The listing builds one solid part. Answer for the finished solid, in the listing's coordinates (mm). A direction names the side the tool comes from. Coordinates: 2 decimals unless noted, no trailing zeros. Write each loop counter-clockwise with the first axis right and the second up, starting at its lowest first coordinate (ties: lowest second). Pieces come first, ordered by that corner, then holes.
from build123d import *

# Parameters (mm, degrees)
F0_R     = 3
F0_W     = 19
F0_H     = 1.5
F0_R_2   = 1
F0_W_2   = 1.5
F0_H_2   = 17.5
F0_H_3   = 11.5
F0_W_3   = 11.5
F0_W_4   = 8.5
F0_W_5   = 4.1
F1_DEPTH = 1.5
F2_DEPTH = 3
F3_DEPTH = 8
F4_DEPTH = 4.5
F5_R     = 1
F6_DEPTH = 1.5


with BuildPart() as f1:
    # F0 (on Top) → F1 (new body)
    with BuildSketch(Plane.XY):
        with BuildLine():
            Line((29.7, 15.2), (-29.7, 15.2))
            ThreePointArc((-29.7, 15.2), (-31.8213203436, 14.3213203436), (-32.7, 12.2))
            Line((-32.7, 12.2), (-32.7, 7.65))
            Line((-32.7, 7.65), (-32.7, -3.85))
            Line((-32.7, -3.85), (-32.7, -12.2))
            ThreePointArc((-32.7, -12.2), (-31.8213203436, -14.3213203436), (-29.7, -15.2))
            Line((-29.7, -15.2), (-25.85, -15.2))
            Line((-25.85, -15.2), (-14.35, -15.2))
            Line((-14.35, -15.2), (4.65, -15.2))
            Line((4.65, -15.2), (13.15, -15.2))
            Line((13.15, -15.2), (17.25, -15.2))
            Line((17.25, -15.2), (25.75, -15.2))
            Line((25.75, -15.2), (29.7, -15.2))
            ThreePointArc((29.7, -15.2), (31.8213203436, -14.3213203436), (32.7, -12.2))
            Line((32.7, -12.2), (32.7, -8.75))
            Line((32.7, -8.75), (32.7, 8.75))
            Line((32.7, 8.75), (32.7, 12.2))
            ThreePointArc((32.7, 12.2), (31.8213203436, 14.3213203436), (29.7, 15.2))
        make_face()
        with Locations((-29, -11.5)):
            Circle(F0_R, mode=Mode.SUBTRACT)
        with Locations((29, -11.5)):
            Circle(F0_R, mode=Mode.SUBTRACT)
        with Locations((-29, 11.5)):
            Circle(F0_R, mode=Mode.SUBTRACT)
        with Locations((29, 11.5)):
            Circle(F0_R, mode=Mode.SUBTRACT)
        with BuildLine():
            ThreePointArc((-32.7, 12.2), (-31.8213203436, 14.3213203436), (-29.7, 15.2))
            Line((-29.7, 15.2), (29.7, 15.2))
            ThreePointArc((29.7, 15.2), (31.8213203436, 14.3213203436), (32.7, 12.2))
            Line((32.7, 12.2), (32.7, 8.75))
            Line((32.7, 8.75), (34.2, 8.75))
            Line((34.2, 8.75), (34.2, 13.7))
            ThreePointArc((34.2, 13.7), (33.3213203436, 15.8213203436), (31.2, 16.7))
            Line((31.2, 16.7), (-31.2, 16.7))
            ThreePointArc((-31.2, 16.7), (-33.3213203436, 15.8213203436), (-34.2, 13.7))
            Line((-34.2, 13.7), (-34.2, 7.65))
            Line((-34.2, 7.65), (-32.7, 7.65))
            Line((-32.7, 7.65), (-32.7, 12.2))
        make_face()
        with BuildLine():
            Line((-32.7, -12.2), (-32.7, -3.85))
            Line((-32.7, -3.85), (-34.2, -3.85))
            Line((-34.2, -3.85), (-34.2, -13.7))
            ThreePointArc((-34.2, -13.7), (-33.3213203436, -15.8213203436), (-31.2, -16.7))
            Line((-31.2, -16.7), (-25.85, -16.7))
            Line((-25.85, -16.7), (-25.85, -15.2))
            Line((-25.85, -15.2), (-29.7, -15.2))
            ThreePointArc((-29.7, -15.2), (-31.8213203436, -14.3213203436), (-32.7, -12.2))
        make_face()
        with Locations((-4.85, -15.95)):
            Rectangle(F0_W, F0_H)
        with Locations((-29, -11.5)):
            Circle(F0_R)
        with Locations((-29, -11.5)):
            Circle(F0_R_2, mode=Mode.SUBTRACT)
        with Locations((-29, 11.5)):
            Circle(F0_R)
        with Locations((-29, 11.5)):
            Circle(F0_R_2, mode=Mode.SUBTRACT)
        with Locations((29, -11.5)):
            Circle(F0_R)
        with Locations((29, -11.5)):
            Circle(F0_R_2, mode=Mode.SUBTRACT)
        with Locations((29, 11.5)):
            Circle(F0_R)
        with Locations((29, 11.5)):
            Circle(F0_R_2, mode=Mode.SUBTRACT)
        with Locations((33.45, 0)):
            Rectangle(F0_W_2, F0_H_2)
        with BuildLine():
            Line((34.2, -8.75), (32.7, -8.75))
            Line((32.7, -8.75), (32.7, -12.2))
            ThreePointArc((32.7, -12.2), (31.8213203436, -14.3213203436), (29.7, -15.2))
            Line((29.7, -15.2), (25.75, -15.2))
            Line((25.75, -15.2), (25.75, -16.7))
            Line((25.75, -16.7), (31.2, -16.7))
            ThreePointArc((31.2, -16.7), (33.3213203436, -15.8213203436), (34.2, -13.7))
            Line((34.2, -13.7), (34.2, -8.75))
        make_face()
        with Locations((-33.45, 1.9)):
            Rectangle(F0_W_2, F0_H_3)
        with Locations((-20.1, -15.95)):
            Rectangle(F0_W_3, F0_H)
        with Locations((21.5, -15.95)):
            Rectangle(F0_W_4, F0_H)
        with Locations((8.9, -15.95)):
            Rectangle(F0_W_4, F0_H)
        with Locations((15.2, -15.95)):
            Rectangle(F0_W_5, F0_H)
        with Locations((-29, -11.5)):
            Circle(F0_R_2)
        with Locations((-29, 11.5)):
            Circle(F0_R_2)
        with Locations((29, -11.5)):
            Circle(F0_R_2)
        with Locations((29, 11.5)):
            Circle(F0_R_2)
    extrude(amount=-F1_DEPTH)

    # F0 (on Top) → F2 (join)
    with BuildSketch(Plane.XY):
        with Locations((-29, 11.5)):
            Circle(F0_R)
        with Locations((-29, 11.5)):
            Circle(F0_R_2, mode=Mode.SUBTRACT)
        with Locations((-29, -11.5)):
            Circle(F0_R)
        with Locations((-29, -11.5)):
            Circle(F0_R_2, mode=Mode.SUBTRACT)
        with Locations((29, 11.5)):
            Circle(F0_R)
        with Locations((29, 11.5)):
            Circle(F0_R_2, mode=Mode.SUBTRACT)
        with Locations((29, -11.5)):
            Circle(F0_R)
        with Locations((29, -11.5)):
            Circle(F0_R_2, mode=Mode.SUBTRACT)
    extrude(amount=F2_DEPTH)

    # F0 (on Top) → F3 (join)
    with BuildSketch(Plane.XY):
        with BuildLine():
            Line((-32.7, -12.2), (-32.7, -3.85))
            Line((-32.7, -3.85), (-34.2, -3.85))
            Line((-34.2, -3.85), (-34.2, -13.7))
            ThreePointArc((-34.2, -13.7), (-33.3213203436, -15.8213203436), (-31.2, -16.7))
            Line((-31.2, -16.7), (-25.85, -16.7))
            Line((-25.85, -16.7), (-25.85, -15.2))
            Line((-25.85, -15.2), (-29.7, -15.2))
            ThreePointArc((-29.7, -15.2), (-31.8213203436, -14.3213203436), (-32.7, -12.2))
        make_face()
        with BuildLine():
            ThreePointArc((-32.7, 12.2), (-31.8213203436, 14.3213203436), (-29.7, 15.2))
            Line((-29.7, 15.2), (29.7, 15.2))
            ThreePointArc((29.7, 15.2), (31.8213203436, 14.3213203436), (32.7, 12.2))
            Line((32.7, 12.2), (32.7, 8.75))
            Line((32.7, 8.75), (34.2, 8.75))
            Line((34.2, 8.75), (34.2, 13.7))
            ThreePointArc((34.2, 13.7), (33.3213203436, 15.8213203436), (31.2, 16.7))
            Line((31.2, 16.7), (-31.2, 16.7))
            ThreePointArc((-31.2, 16.7), (-33.3213203436, 15.8213203436), (-34.2, 13.7))
            Line((-34.2, 13.7), (-34.2, 7.65))
            Line((-34.2, 7.65), (-32.7, 7.65))
            Line((-32.7, 7.65), (-32.7, 12.2))
        make_face()
        with Locations((-4.85, -15.95)):
            Rectangle(F0_W, F0_H)
        with Locations((15.2, -15.95)):
            Rectangle(F0_W_5, F0_H)
        with BuildLine():
            Line((34.2, -8.75), (32.7, -8.75))
            Line((32.7, -8.75), (32.7, -12.2))
            ThreePointArc((32.7, -12.2), (31.8213203436, -14.3213203436), (29.7, -15.2))
            Line((29.7, -15.2), (25.75, -15.2))
            Line((25.75, -15.2), (25.75, -16.7))
            Line((25.75, -16.7), (31.2, -16.7))
            ThreePointArc((31.2, -16.7), (33.3213203436, -15.8213203436), (34.2, -13.7))
            Line((34.2, -13.7), (34.2, -8.75))
        make_face()
    extrude(amount=F3_DEPTH)

    # F0 (on Top) → F4 (join)
    with BuildSketch(Plane.XY):
        with Locations((-33.45, 1.9)):
            Rectangle(F0_W_2, F0_H_3)
        with Locations((-20.1, -15.95)):
            Rectangle(F0_W_3, F0_H)
        with Locations((8.9, -15.95)):
            Rectangle(F0_W_4, F0_H)
        with Locations((21.5, -15.95)):
            Rectangle(F0_W_4, F0_H)
        with Locations((33.45, 0)):
            Rectangle(F0_W_2, F0_H_2)
    extrude(amount=F4_DEPTH)

    # F5 (on Top) → F6 (join)
    with BuildSketch(Plane.XY):
        with BuildLine():
            Line((28.2029380615, -16.7), (-28.2029380615, -16.7))
            Line((-28.2029380615, -16.7), (-25.7184552477, -23.52606043))
            ThreePointArc((-25.7184552477, -23.52606043), (-25.0528877677, -24.5886342507), (-24.0111634719, -25.2863832647))
            ThreePointArc((-24.0111634719, -25.2863832647), (-24.3642014734, -20.9050168641), (-20.5, -23))
            ThreePointArc((-20.5, -23), (-21.215336344, -24.7507071813), (-22.9519805079, -25.4995387831))
            ThreePointArc((-22.9519805079, -25.4995387831), (-22.9256799576, -25.4998846936), (-22.8993773854, -25.5))
            Line((-22.8993773854, -25.5), (22.8993773854, -25.5))
            ThreePointArc((22.8993773854, -25.5), (22.9256799576, -25.4998846936), (22.9519805079, -25.4995387831))
            ThreePointArc((22.9519805079, -25.4995387831), (21.2492928187, -21.215336344), (25.5, -23))
            ThreePointArc((25.5, -23), (25.0949831359, -24.3642014734), (24.0111634719, -25.2863832647))
            ThreePointArc((24.0111634719, -25.2863832647), (25.0528877677, -24.5886342507), (25.7184552477, -23.52606043))
            Line((25.7184552477, -23.52606043), (28.2029380615, -16.7))
        make_face()
        with BuildLine():
            ThreePointArc((-20.5, -23), (-24.3642014734, -20.9050168641), (-24.0111634719, -25.2863832647))
            ThreePointArc((-24.0111634719, -25.2863832647), (-23.4912467766, -25.441035638), (-22.9519805079, -25.4995387831))
            ThreePointArc((-22.9519805079, -25.4995387831), (-21.215336344, -24.7507071813), (-20.5, -23))
        make_face()
        with Locations((-23, -23)):
            Circle(F5_R, mode=Mode.SUBTRACT)
        with BuildLine():
            ThreePointArc((22.9519805079, -25.4995387831), (23.4912467766, -25.441035638), (24.0111634719, -25.2863832647))
            ThreePointArc((24.0111634719, -25.2863832647), (25.0949831359, -24.3642014734), (25.5, -23))
            ThreePointArc((25.5, -23), (21.2492928187, -21.215336344), (22.9519805079, -25.4995387831))
        make_face()
        with Locations((23, -23)):
            Circle(F5_R, mode=Mode.SUBTRACT)
        with BuildLine():
            Line((-25.7184552477, 23.52606043), (-28.2029380615, 16.7))
            Line((-28.2029380615, 16.7), (28.2029380615, 16.7))
            Line((28.2029380615, 16.7), (25.7184552477, 23.52606043))
            ThreePointArc((25.7184552477, 23.52606043), (25.0528877677, 24.5886342507), (24.0111634719, 25.2863832647))
            ThreePointArc((24.0111634719, 25.2863832647), (25.0949831359, 24.3642014734), (25.5, 23))
            ThreePointArc((25.5, 23), (21.2492928187, 21.215336344), (22.9519805079, 25.4995387831))
            ThreePointArc((22.9519805079, 25.4995387831), (22.9256799576, 25.4998846936), (22.8993773854, 25.5))
            Line((22.8993773854, 25.5), (-22.8993773854, 25.5))
            ThreePointArc((-22.8993773854, 25.5), (-22.9256799576, 25.4998846936), (-22.9519805079, 25.4995387831))
            ThreePointArc((-22.9519805079, 25.4995387831), (-21.215336344, 24.7507071813), (-20.5, 23))
            ThreePointArc((-20.5, 23), (-24.3642014734, 20.9050168641), (-24.0111634719, 25.2863832647))
            ThreePointArc((-24.0111634719, 25.2863832647), (-25.0528877677, 24.5886342507), (-25.7184552477, 23.52606043))
        make_face()
        with BuildLine():
            ThreePointArc((-22.9519805079, 25.4995387831), (-23.4912467766, 25.441035638), (-24.0111634719, 25.2863832647))
            ThreePointArc((-24.0111634719, 25.2863832647), (-24.3642014734, 20.9050168641), (-20.5, 23))
            ThreePointArc((-20.5, 23), (-21.215336344, 24.7507071813), (-22.9519805079, 25.4995387831))
        make_face()
        with Locations((-23, 23)):
            Circle(F5_R, mode=Mode.SUBTRACT)
        with BuildLine():
            ThreePointArc((25.5, 23), (25.0949831359, 24.3642014734), (24.0111634719, 25.2863832647))
            ThreePointArc((24.0111634719, 25.2863832647), (23.4912467766, 25.441035638), (22.9519805079, 25.4995387831))
            ThreePointArc((22.9519805079, 25.4995387831), (21.2492928187, 21.215336344), (25.5, 23))
        make_face()
        with Locations((23, 23)):
            Circle(F5_R, mode=Mode.SUBTRACT)
    extrude(amount=-F6_DEPTH)


solid = f1.part
Q1. The part is cut by section C-C, the plane z = 6.25. State how many separate pieces and enclosed holes the cut face has, then the cut area to 3 significant figures.
Answers below:
separate pieces: 5
enclosed holes: 0
area: 210 mm2
Q2. The part is cut by section D-D, the plane x = 15. Write down the section's boundary in (y, z).
Answers below:
outline: (-25.5, -1.5) - (25.5, -1.5) - (25.5, 0) - (16.7, 0) - (16.7, 8) - (15.2, 8) - (15.2, 0) - (-15.2, 0) - (-15.2, 8) - (-16.7, 8) - (-16.7, 0) - (-25.5, 0) - close
Q3. Find the intervals of material crossed by probe 1 along Y at (x, z) = (-23, -0.45); probe 2 along X at (y, z) = (5.5, 1.5); probe 3 along Y at (x, z) = (29, 3.25), in increasing order.
Answers below:
probe 1: y = -25.5 to -24, -22 to 22, 24 to 25.5
probe 2: x = -34.2 to -32.7, 32.7 to 34.2
probe 3: y = -16.7 to -15.2, 15.2 to 16.7
Q4. Which of the six approach directions +Z, -Z, +X, -X, +Y, -Y give full straight-line access (tool end or side, diameter ignored) to faces 4 (the face through (25.75, -16, 6)), 5 (the face through (-29, 10, 3)), 6 (the face through (33, 8.75, 6))?
Answers below:
face 4: +Z, -Y
face 5: +Z
face 6: +Z, +X
Q5. The part is cut by section B-B, the plane x = 29. Write down the section's boundary in (y, z), then the cut area to 3 significant figures.
Answers below:
outline: (-16.7, -1.5) - (16.7, -1.5) - (16.7, 8) - (15.2, 8) - (15.2, 0) - (14.5, 0) - (14.5, 3) - (12.5, 3) - (12.5, 0) - (10.5, 0) - (10.5, 3) - (8.5, 3) - (8.5, 0) - (-8.5, 0) - (-8.5, 3) - (-10.5, 3) - (-10.5, 0) - (-12.5, 0) - (-12.5, 3) - (-14.5, 3) - (-14.5, 0) - (-15.2, 0) - (-15.2, 8) - (-16.7, 8) - close
area: 98.1 mm2
Q6. Given pin 1 (0.6 mm diameter, centred on x = -29, y = 11.5, fed in from +Z); pin 2 (3 mm diameter, centred on x = -29, y = 11.5, fed in from +Z); pin 3 (3 mm diameter, centred on x = 1, z = 2, fed in from -Y), each flat-ended and moving along its own axis, determine where each tip first touches the part or whether it passes through.
Answers below:
pin 1: stops at z = 0
pin 2: stops at z = 3
pin 3: stops at y = -16.7
Q7. Determine the mould class of faces 1 (the face through (-33, -3.85, 6)), 2 (the face through (-32, 11.6, 1.5)), 3 (the face through (34.2, 0, 2)) for opening direction X: released by +X, released by -X, zero draft, split by the parting line, or undercut.
Answers below:
face 1: zero draft
face 2: undercut
face 3: released by +X
Q8. The part is cut by section A-A, the plane y = -11.5. Write down the section's boundary in (x, z), then the cut area to 3 significant figures.
Answers below:
outline: (-34.2, -1.5) - (34.2, -1.5) - (34.2, 8) - (32.7, 8) - (32.7, 0) - (32, 0) - (32, 3) - (30, 3) - (30, 0) - (28, 0) - (28, 3) - (26, 3) - (26, 0) - (-26, 0) - (-26, 3) - (-28, 3) - (-28, 0) - (-30, 0) - (-30, 3) - (-32, 3) - (-32, 0) - (-32.7, 0) - (-32.7, 8) - (-34.2, 8) - close
area: 151 mm2
